```python
from build123d import *

# Parameters (mm, degrees)
SKETCH1_R           = 3.45
BOSS_EXTRUDE1_DEPTH = 3
SKETCH2_R           = 5.144351969
BOSS_EXTRUDE2_DEPTH = 5
BOSS_EXTRUDE2_TAPER = 3
BOSS_EXTRUDE3_DEPTH = 0.5
CIRPATTERN1_COUNT   = 18
SKETCH5_R           = 4.5
BOSS_EXTRUDE5_DEPTH = 0.5


with BuildPart() as part:
    # Sketch1 → Boss-Extrude1 (new body)
    with BuildSketch(Plane(origin=(0, 0, 0), x_dir=(1, 0, 0), z_dir=(0, 1, 0))):
        with Locations(Location((0, 0, 0), (0, 0, 270))):
            Circle(SKETCH1_R)
    extrude(amount=BOSS_EXTRUDE1_DEPTH)

    # Sketch2 → Boss-Extrude2 (add)
    with BuildSketch(Plane(origin=(0, 3, 0), x_dir=(1, 0, 0), z_dir=(0, 1, 0))):
        Circle(SKETCH2_R)
    extrude(amount=BOSS_EXTRUDE2_DEPTH, taper=BOSS_EXTRUDE2_TAPER)

    # Sketch4 → Boss-Extrude3 (add, symmetric)
    with BuildSketch(Plane.XY):
        Polygon((-4.498373747, 8.334987069), (-4.806833662, 2.602773665), (-5.552278454, 2.602773665), (-5.24381854, 8.334987069), align=None)
    boss_extrude3 = extrude(amount=BOSS_EXTRUDE3_DEPTH, both=True)

    # CirPattern1: Boss-Extrude3 ×18 about axis
    cirpattern1_axis = Axis((0, 0, 0), (0, 1, 0))
    for i in range(1, CIRPATTERN1_COUNT):
        add(boss_extrude3.rotate(cirpattern1_axis, i * 360 / CIRPATTERN1_COUNT))

    # Sketch5 → Boss-Extrude5 (add)
    with BuildSketch(Plane(origin=(0, 8, 0), x_dir=(1, 0, 0), z_dir=(0, 1, 0))):
        with Locations(Location((0, 0, 0), (0, 0, 270))):
            Circle(SKETCH5_R)
    extrude(amount=BOSS_EXTRUDE5_DEPTH)


solid = part.part
```
CAD build for the part. Positions are in the model's coordinates, mm. A direction names the side the tool comes from. Coordinates: 2 decimals unless noted, no trailing zeros. Order: outer loops, then holes, each group sorted by start corner. A loop starts at its lowest first (then second) coordinate and runs counter-clockwise, first axis right, second up. Notation, with made-up numbers: (42.25, 10) -> (49.25, 10) arc R24 cw to (49.25, 24) -> close; hole circle Ø7 at (-1.5, 36). An arc over 180 degrees is marked (long way). Use one line per item in the form item = value. Start each with the question number.
1) Pull direction Z, two halves, no side cores. Call faces 1 (the flat face through (-0.4, 6.15, -5.14)), 2 (the flat face through (-0.4, 6.15, 5.14)), 3 (the flat face through (-0.8, 8.335, 4.8)), 4 (the flat face through (-1.384, 6.146, 4.97)): +Z half, -Z half, draft (parallel to the pull), parting line (faces both ways), or undercut.
2) Drill centre lines: L1, parallel to X at y = 2.75, z = 0.25; L2, parallel to Y at x = -3.75, z = -1.25; L3, parallel to Y at x = 0.25, z = -4.75. Where is each one in solid material? Low to high. Write a range as [from, to].
3) Band-saw the part on A-A on x = 0. Give the cut face in (y, z).
4) Band-saw the part on B-B on y = 2.25. Give the cut face in (x, z), then the cut area to 3 significant figures.
5) Drop flat-ended pins along their axis: pin 1 (0.8 mm diameter, centred on x = -5, z = -2, fed in from -Y); pin 2 (1.1 mm diameter, centred on x = -5, z = -1.5, fed in from +Y) (3 decimals); pin 3 (3 mm diameter, centred on y = 5, z = 3, fed in from +X). Give the stop position or say it passes through.
6) Tool access for faces 5 (the flat face through (4, 8.335, -3)), 6 (the flat face through (-2.6, 2.603, 4.5)), 7 (the flat face through (2.6, 2.603, -4.5)), 8 (the flat face through (5, 2.603, -2)), 9 (the flat face through (-5.4, 5.4, 0)): list every direction of +Z, -Z, +X, -X, +Y, -Y with a clear straight run to the whole face (end or side of a thin tool).
Entries:
q1.face_1 = -Z half
q1.face_2 = +Z half
q1.face_3 = draft
q1.face_4 = undercut
q2.L1 = [-5.54, -4.8], [-3.44, 3.44], [4.8, 5.54]
q2.L2 = [3, 8.5]
q2.L3 = [3, 8]
q3.outline = (0, -3.45) -> (3, -3.45) -> (3, -5.14) -> (8, -4.88) -> (8, -4.5) -> (8.5, -4.5) -> (8.5, 4.5) -> (8, 4.5) -> (8, 4.88) -> (3, 5.14) -> (3, 3.45) -> (0, 3.45) -> close
q4.outline = circle Ø6.9 at (0, 0)
q4.area = 37.4 mm2
q5.pin_1 = 2.6
q5.pin_2 = 8.335
q5.pin_3 = 5.23
q6.face_5 = -Z, +X, +Y
q6.face_6 = +Z, +X, -X, -Y
q6.face_7 = -Z, +X, -X, -Y
q6.face_8 = +Z, -Z, +X, -Y
q6.face_9 = +Z, -Z, -X, +Y
